Read the model definition and answer for the solid it produces. Units are mm, in the model's axes. A direction names the side the tool comes from. Coordinates: 2 decimals unless noted, no trailing zeros. Loops run counter-clockwise (first coordinate to the right, second up) from the corner with the lowest first, then second, coordinate; pieces in that order, holes last. Notation, with made-up numbers: (-8.5, -38.75) -> (17.5, -38.75) arc R27 ccw to (17.5, -22.75) -> close; hole circle Ø8 at (50, 3.5). An arc over 180 degrees is marked (long way). Answer as a JSON object with one key per item and string values. Group by question number.
Q1. Each of these flat-tipped pins is pushed along its axis until it touches: P1, Ø0.5, axis at x = 24.5, z = 2, coming from the +Y side; P2, Ø2, axis at x = -19.5, z = 1, coming from the +Y side; P3, Ø1.5, axis at x = 13, y = 4, coming from the -Z side; P4, Ø2, axis at x = 9.5, y = 1.5, coming from the +Z side. Where does it stop, or does it pass through?
Q2. The part is cut by section B-B on x = -0.5. Write down the section's boundary in (y, z).
Q3. For faces 4 (the flat face through (-17, 3, 0)), 5 (the flat face through (0, 7, 0)), 6 (the flat face through (-8, 6, 0)), 7 (the flat face through (0, 4, 1)), 8 (the flat face through (2.25, 2, 1)), determine the directions among +Z, -Z, +X, -X, +Y, -Y from which every point of the face is accessible in a straight line to the end or side of a thin tool.
Q4. Straight lines are drawn through the part: line 1 along X through (y, z) = (4.5, 4.25); line 2 along X through (y, z) = (3.25, -4.75); line 3 along X through (y, z) = (0.75, 6.25). For each, find the intervals that lie inside material, in ascending order. Write a range as [from, to].
Q5. Determine the mould class of faces 1 (the flat face through (24.5, 6, 0.1)), 2 (the flat face through (24, 4, 0)), 3 (the flat face through (0, 2, -7.2)) for opening direction Y: released by +Y, released by -Y, zero draft, split by the parting line, or undercut.
Q6. The part is cut by section D-D on y = 2. Write down the section's boundary in (x, z), and give its area (3 significant figures).
Q7. The part is cut by section A-A on y = 5. Write down the section's boundary in (x, z).
from build123d import *

# Parameters (mm, degrees)
SKETCH1_W           = 15
SKETCH1_H           = 18
BOSS_EXTRUDE1_DEPTH = 7
CUT_EXTRUDE1_DEPTH  = 16.2
SKETCH9_W           = 16
SKETCH9_H           = 6
BOSS_EXTRUDE2_DEPTH = 18
SKETCH13_W          = 16
SKETCH13_H          = 6
BOSS_EXTRUDE3_DEPTH = 18
SKETCH14_W          = 15
SKETCH14_H          = 3
CUT_EXTRUDE5_DEPTH  = 32.55
FILLET1_R           = 0.5


with BuildPart() as part:
    # Sketch1 → Boss-Extrude1 (new body)
    with BuildSketch(Plane(origin=(0, 0, 0), x_dir=(1, 0, 0), z_dir=(0, 1, 0))):
        Rectangle(SKETCH1_W, SKETCH1_H)
    extrude(amount=BOSS_EXTRUDE1_DEPTH)

    # Sketch2 → Cut-Extrude1 (cut)
    with BuildSketch(Plane.XY.offset(9)):
        Polygon((-2.25, 2.6), (-2.25, 0), (2.25, 0), (2.25, 2.6), (4.45, 2.6), (4.45, 4), (-4.45, 4), (-4.45, 2.6), align=None)
    extrude(amount=-CUT_EXTRUDE1_DEPTH, mode=Mode.SUBTRACT)

    # Sketch9 → Boss-Extrude2 (add)
    with BuildSketch(Plane.ZY.offset(7.5)):
        with Locations((0, 3)):
            Rectangle(SKETCH9_W, SKETCH9_H)
    extrude(amount=BOSS_EXTRUDE2_DEPTH)

    # Sketch13 → Boss-Extrude3 (add)
    with BuildSketch(Plane(origin=(7.5, 0, 0), x_dir=(0, 0, -1), z_dir=(1, 0, 0))):
        with Locations((0, 3)):
            Rectangle(SKETCH13_W, SKETCH13_H)
    extrude(amount=BOSS_EXTRUDE3_DEPTH)

    # Sketch14 → Cut-Extrude5 (cut)
    with BuildSketch(Plane.XY.offset(9)):
        with Locations((16.5, 4.5)):
            Rectangle(SKETCH14_W, SKETCH14_H)
        with Locations((-16.5, 4.5)):
            Rectangle(SKETCH14_W, SKETCH14_H)
    extrude(amount=-CUT_EXTRUDE5_DEPTH, mode=Mode.SUBTRACT)

    # Fillet1
    fillet1_edges = [part.edges().sort_by_distance(p)[0] for p in [
        (-7.5, 7, 0),
        (4.875, 0, 9),
        (0, 7, 9),
        (-2.25, 0, 0.9),
        (2.25, 0, 0.9),
        (-7.5, 0, 8.5),
        (-25.5, 6, 0),
        (7.5, 7, 0),
        (-4.875, 0, 9),
        (-7.5, 0, -8.5),
        (0, 0, -9),
        (7.5, 0, -8.5),
        (7.5, 0, 8.5),
        (25.5, 6, 0),
        (7.5, 3.5, 9),
        (-7.5, 3.5, 9),
        (-7.5, 3.5, -9),
        (7.5, 3.5, -9),
        (9, 6, 0),
        (0, 7, -9),
        (-9, 6, 0),
    ]]
    fillet(fillet1_edges, radius=FILLET1_R)


solid = part.part
Final values:
{
 "1": {"P1": "stops at y = 6", "P2": "stops at y = 3", "P3": "passes through", "P4": "stops at z = 8"},
 "2": {"outline": "(0, -8.5) arc R0.5 ccw to (0.5, -9) -> (6.5, -9) arc R0.5 ccw to (7, -8.5) -> (7, 8.5) arc R0.5 ccw to (6.5, 9) -> (4, 9) -> (4, -7.2) -> (0, -7.2) -> close"},
 "3": {"face 4": "+Z, -Z, +Y", "face 5": "+Z, -Z, +X, -X, +Y", "face 6": "+Z, -Z, -X, +Y", "face 7": "+Z", "face 8": "+Z, -Y"},
 "4": {"line 1": "x = [-25.5, -24], [-9, 9], [24, 25.5]", "line 2": "x = [-25.5, -24], [-9, -4.45], [4.45, 9], [24, 25.5]", "line 3": "x = [-25.5, -2.25], [2.25, 25.5]"},
 "5": {"face 1": "released by +Y", "face 2": "zero draft", "face 3": "undercut"},
 "6": {"outline": "(-25.5, -8) -> (-7.5, -8) -> (-7.5, -8.5) arc R0.5 ccw to (-7, -9) -> (7, -9) arc R0.5 ccw to (7.5, -8.5) -> (7.5, -8) -> (25.5, -8) -> (25.5, 8) -> (7.5, 8) -> (7.5, 8.5) arc R0.5 ccw to (7, 9) -> (2.25, 9) -> (2.25, -7.2) -> (-2.25, -7.2) -> (-2.25, 9) -> (-7, 9) arc R0.5 ccw to (-7.5, 8.5) -> (-7.5, 8) -> (-25.5, 8) -> close", "area": "773 mm2"},
 "7": {"outline": "(-25.5, -8) -> (-24, -8) -> (-24, 8) -> (-25.5, 8) -> close; (-9, -8) -> (-7.5, -8) -> (-7.5, -8.5) arc R0.5 ccw to (-7, -9) -> (7, -9) arc R0.5 ccw to (7.5, -8.5) -> (7.5, -8) -> (9, -8) -> (9, 8) -> (7.5, 8) -> (7.5, 8.5) arc R0.5 ccw to (7, 9) -> (-7, 9) arc R0.5 ccw to (-7.5, 8.5) -> (-7.5, 8) -> (-9, 8) -> close; (24, -8) -> (25.5, -8) -> (25.5, 8) -> (24, 8) -> close"}
}
